Design review of the part built by this model. Coordinates are the model's own, in mm. Coordinates: 2 decimals unless noted, no trailing zeros. Order: outer loops, then holes, each group sorted by start corner. A loop starts at its lowest first (then second) coordinate and runs counter-clockwise, first axis right, second up. Notation, with made-up numbers: (47, 62) -> (76, 62) arc R22 cw to (76, 75) -> close; hole circle Ø10 at (-18, 50.25). An arc over 180 degrees is marked (long way). Write item = value, one per line.
```python
from build123d import *

# Parameters (mm, degrees)
SKETCH1_W           = 107.27
SKETCH1_H           = 30.02
BOSS_EXTRUDE1_DEPTH = 10
SKETCH2_R           = 2.5
BOSS_EXTRUDE2_DEPTH = 30
SKETCH3_W           = 67.27
SKETCH3_H           = 10.02
CUT_EXTRUDE1_DEPTH  = 1


with BuildPart() as part:
    # Sketch1 → Boss-Extrude1 (new body)
    with BuildSketch(Plane(origin=(0, 0, 0), x_dir=(1, 0, 0), z_dir=(0, 1, 0))):
        with Locations((53.635, 15.01)):
            Rectangle(SKETCH1_W, SKETCH1_H)
    extrude(amount=BOSS_EXTRUDE1_DEPTH)

    # Sketch2 → Boss-Extrude2 (add)
    with BuildSketch(Plane.ZY):
        with Locations((-15.01, 5)):
            Circle(SKETCH2_R)
    extrude(amount=BOSS_EXTRUDE2_DEPTH)

    # Sketch3 → Cut-Extrude1 (cut)
    with BuildSketch(Plane(origin=(0, 10, 0), x_dir=(1, 0, 0), z_dir=(0, 1, 0))):
        with Locations((53.635, 15.01)):
            Rectangle(SKETCH3_W, SKETCH3_H)
    extrude(amount=-CUT_EXTRUDE1_DEPTH, mode=Mode.SUBTRACT)


solid = part.part
```
(1) We need section B-B (z = -15.01). Write out the cut boundary in (x, y).
Report:
outline = (-30, 2.5) -> (0, 2.5) -> (0, 0) -> (107.27, 0) -> (107.27, 10) -> (87.27, 10) -> (87.27, 9) -> (20, 9) -> (20, 10) -> (0, 10) -> (0, 7.5) -> (-30, 7.5) -> close
(2) We need section D-D (z = -4.5). Write out the cut boundary in (x, y).
Report:
outline = (0, 0) -> (107.27, 0) -> (107.27, 10) -> (0, 10) -> close
(3) The part is to be moulded in two halves that separate along Z. For faces 1 (the cylindrical face through (-14.79, 5.11, -17.508)), 2 (the flat face through (53, 10, -9)), 3 (the flat face through (53, 5, 0)), 4 (the flat face through (53, 9, -15)), say which applies: released by +Z, released by -Z, zero draft, split by the parting line, or undercut.
Report:
face_1 = split by the parting line
face_2 = zero draft
face_3 = released by +Z
face_4 = undercut
(4) Insertion check: pin 1 (4 mm diameter, centred on x = 59.5, z = -13.5, fed in from +Y); pin 2 (1.1 mm diameter, centred on y = 9.5, z = -16, fed in from -X). Each pin has a flat end and moves straight along its axis. Give the tip position at first contact, or say it passes through.
Report:
pin_1 = 9
pin_2 = 0
(5) We need section C-C (x = 76). Write out the cut boundary in (y, z), and give its area (3 significant figures).
Report:
outline = (0, -30.02) -> (10, -30.02) -> (10, -20.02) -> (9, -20.02) -> (9, -10) -> (10, -10) -> (10, 0) -> (0, 0) -> close
area = 290 mm²
(6) We need section A-A (y = 5). Write out the cut boundary in (x, z), and give its area (3 significant figures).
Report:
outline = (-30, -17.51) -> (0, -17.51) -> (0, -30.02) -> (107.27, -30.02) -> (107.27, 0) -> (0, 0) -> (0, -12.51) -> (-30, -12.51) -> close
area = 3,370 mm²
(7) For L1, parallel to X at y = 1.5, z = -27.5; L2, parallel to Y at x = 52, z = -13; L3, parallel to Z at x = -17, y = 4.25, list the stretches that pass through material, from the lowest coordinate up.
Report:
L1 = 0 to 107.27
L2 = 0 to 9
L3 = -17.39 to -12.63
